Here's the drawing with two shaded views (mm, measured from the low corner). I have some questions. Coordinates: 2 decimals unless noted, no trailing zeros. Order: outer loops, then holes, each group sorted by start corner. A loop starts at its lowest first (then second) coordinate and runs counter-clockwise, first axis right, second up. Notation, with made-up numbers: M 39,31.5 L 53,31.5 A28 cw 53,54.5 Z; hole C -34.5,-29.75 d10. An arc over 180 degrees is marked long. Put each result on its own line as item: value. Start each with the question number.
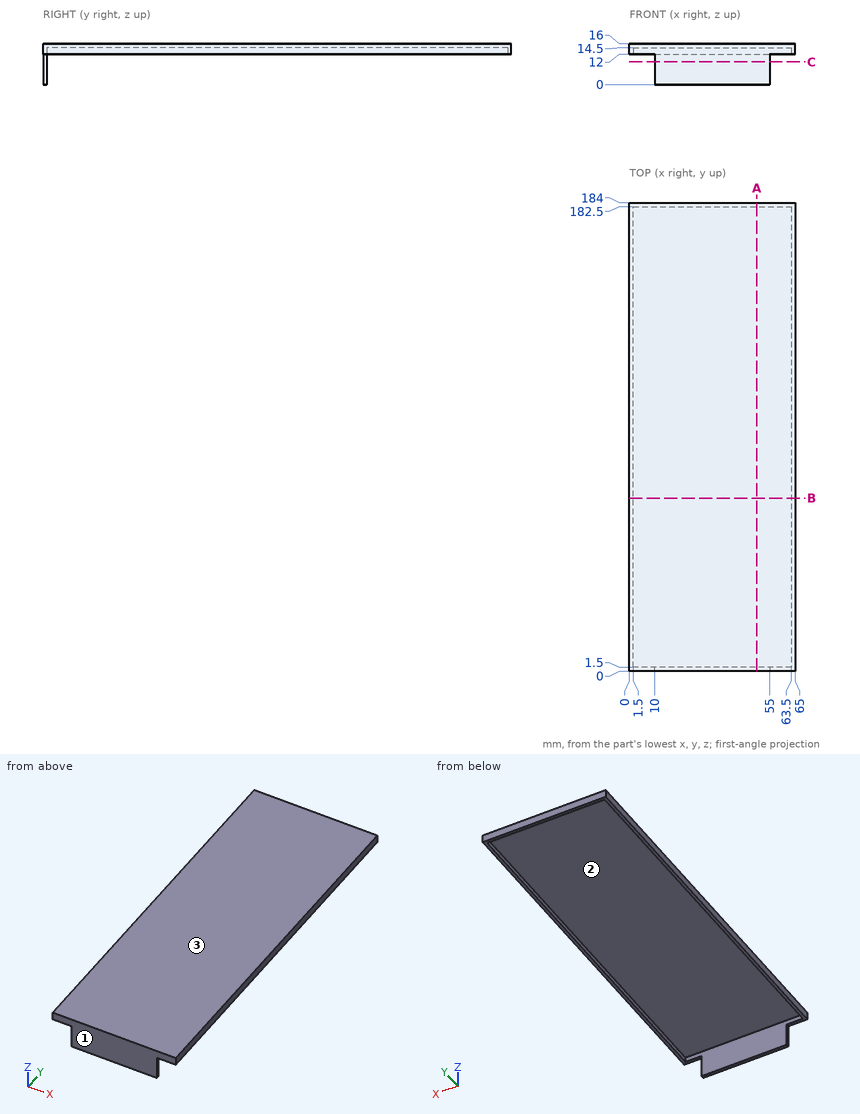
Item 1: For pin 1 Ø1.6 at (y, z) = (0.5, 6.5) entering from -X; pin 2 Ø6 at (x, y) = (43, 162.5) entering from -Z; pin 3 Ø5 at (x, z) = (36.5, 7.5) entering from +Y, each with a flat end and sliding along its axis, tell me the tip position at first contact or that it passes through.
Item 2: If we section it at C-C on z = 9: Write out the boundary of the cut face in (x, y), then the cut area to 3 significant figures.
Item 3: If we section it at B-B on y = 68: Write out the boundary of the cut face in (x, z), then the cut area to 3 significant figures.
Item 4: If we mould it in two halves opening along Y, with no side actions, what happens to the marked faces 1, 2 and 3? For each: released by +Y, released by -Y, zero draft, split by the parting line, or undercut.
Item 5: I need wall thicknesses on probe 1 along X at (y, z) = (141.5, 13); probe 2 along Y at (x, z) = (44, 13); probe 3 along Z at (x, y) = (32.5, 130). Which ranges of each line are inside material? Lowest first, please.
Item 6: If we section it at A-A on x = 50: Write out the boundary of the cut face in (y, z).
Geometry check:
1. pin 1: stops at x = 10
1. pin 2: stops at z = 14.5
1. pin 3: stops at y = 1.5
2. outline: M 10,0 L 55,0 L 55,1.5 L 10,1.5 Z
2. area: 67.5 mm²
3. outline: M 0,12 L 1.5,12 L 1.5,14.5 L 63.5,14.5 L 63.5,12 L 65,12 L 65,16 L 0,16 Z
3. area: 105 mm²
4. face 1: released by -Y
4. face 2: undercut
4. face 3: zero draft
5. probe 1: x = 0 to 1.5, 63.5 to 65
5. probe 2: y = 0 to 1.5, 182.5 to 184
5. probe 3: z = 14.5 to 16
6. outline: M 0,0 L 1.5,0 L 1.5,14.5 L 182.5,14.5 L 182.5,12 L 184,12 L 184,16 L 0,16 Z
